```python
from build123d import *

# Parameters (mm, degrees)
SKETCH1_W                                        = 30
SKETCH1_H                                        = 30
BOSS_EXTRUDE1_DEPTH                              = 11
CUT_EXTRUDE1_DEPTH                               = 1.55
CUT_EXTRUDE2_DEPTH                               = 31.712375356
SKETCH7_W                                        = 5.55
SKETCH7_H                                        = 1.8
CUT_EXTRUDE3_DEPTH                               = 5.55
CBORE_FOR_M3_HEX_HEAD_MACHINE_SCREW1_D           = 3.5
CBORE_FOR_M3_HEX_HEAD_MACHINE_SCREW1_CBORE_D     = 6.5
CBORE_FOR_M3_HEX_HEAD_MACHINE_SCREW1_CBORE_DEPTH = 4
SKETCH10_W                                       = 1.7
SKETCH10_H                                       = 12.55
CUT_EXTRUDE4_DEPTH                               = 1.8
CUT_EXTRUDE4_DEPTH_BACK                          = 2
SKETCH14_W                                       = 13
SKETCH14_H                                       = 30


with BuildPart() as part:
    # Sketch1 → Boss-Extrude1 (new body)
    with BuildSketch(Plane(origin=(0, 0, 5), x_dir=(-1, 0, 0), z_dir=(0, 0, -1))):
        Rectangle(SKETCH1_W, SKETCH1_H)
    extrude(amount=-BOSS_EXTRUDE1_DEPTH)

    # Sketch2 → Cut-Extrude1 (cut)
    with BuildSketch(Plane(origin=(0, -4.95, 0), x_dir=(1, 0, 0), z_dir=(0, 1, 0))):
        with BuildLine():
            Line((7.432729441, -5), (-7.432729441, -5))
            ThreePointArc((-7.432729441, -5), (-7.633699531, -5.794473784), (-7.75, -6.605677687))
            Line((-7.75, -6.605677687), (-7.75, -8))
            ThreePointArc((-7.75, -8), (1.508365059, -14.936538374), (7.432729441, -5))
        make_face()
    extrude(amount=-CUT_EXTRUDE1_DEPTH, mode=Mode.SUBTRACT)

    # Sketch3 → Cut-Extrude2 (cut, through all)
    with BuildSketch(Plane(origin=(0, -6.5, 0), x_dir=(-1, 0, 0), z_dir=(0, 1, 0))):
        with BuildLine():
            Line((-5.125, 5), (5.125, 5))
            Line((5.125, 5), (5.125, 8))
            ThreePointArc((5.125, 8), (0, 13.125), (-5.125, 8))
            Line((-5.125, 8), (-5.125, 5))
        make_face()
    extrude(amount=-CUT_EXTRUDE2_DEPTH, mode=Mode.SUBTRACT)

    # Sketch7 → Cut-Extrude3 (cut)
    with BuildSketch(Plane(origin=(0, 0, 5), x_dir=(-1, 0, 0), z_dir=(0, 0, -1))):
        with Locations((0, -1.55)):
            Rectangle(SKETCH7_W, SKETCH7_H)
    extrude(amount=-CUT_EXTRUDE3_DEPTH, mode=Mode.SUBTRACT)

    # CBORE for M3 Hex Head Machine Screw1 (through all)
    with Locations(Plane(origin=(0, 0, 5), x_dir=(-1, 0, 0), z_dir=(0, 0, -1))):
        with Locations((-10, 10), (-10, -10), (10, -10), (10, 10)):
            CounterBoreHole(CBORE_FOR_M3_HEX_HEAD_MACHINE_SCREW1_D / 2, CBORE_FOR_M3_HEX_HEAD_MACHINE_SCREW1_CBORE_D / 2, CBORE_FOR_M3_HEX_HEAD_MACHINE_SCREW1_CBORE_DEPTH)

    # Sketch10 → Ø3.4 (3.4) Diameter Hole1 (revolve, cut)
    with BuildSketch(Plane(origin=(0, -2.45, 8), x_dir=(0, 0, 1), z_dir=(1, 0, 0))):
        with Locations((0.85, 6.275)):
            Rectangle(SKETCH10_W, SKETCH10_H)
    revolve(axis=Axis((0, 3.9, 8), (0, -1, 0)), mode=Mode.SUBTRACT)

    # Sketch12 → CSK for M3 Flat Head Machine Screw1 (revolve, cut)
    with BuildSketch(Plane(origin=(0, 15, 8), x_dir=(0, 0, 1), z_dir=(1, 0, 0))):
        Polygon((0, 0), (0, 30), (1.7, 30), (1.7, 4.931333959), (3.25, 4), (3.25, 0), align=None)
    revolve(axis=Axis((0, 21.35, 8), (0, -1, 0)), mode=Mode.SUBTRACT)

    # Sketch14 → Cut-Extrude4 (cut, two sides: drawn at the far end of the back side and taken through both)
    with BuildSketch(Plane(origin=(0, -6.5, 0), x_dir=(-1, 0, 0), z_dir=(0, 1, 0)).offset(-CUT_EXTRUDE4_DEPTH_BACK)):
        with Locations((-0.068435325, 5)):
            Rectangle(SKETCH14_W, SKETCH14_H)
    extrude(amount=CUT_EXTRUDE4_DEPTH + CUT_EXTRUDE4_DEPTH_BACK, mode=Mode.SUBTRACT)


solid = part.part
```
Could you check a few things on this model? Use its own coordinates, in mm. A direction names the side the tool comes from. Coordinates: 2 decimals unless noted, no trailing zeros. Write each loop counter-clockwise with the first axis right and the second up, starting at its lowest first coordinate (ties: lowest second). Pieces come first, ordered by that corner, then holes. Notation, with made-up numbers: M -19,35 L -11,35 A25 ccw -11,61 Z; hole C -12,62.25 d3. An arc over 180 degrees is marked long. Answer as CSV lines item,"result". Start each with the question number.
1) I want a section at D-D, the plane x = 0. Please give me the cut outline in (y, z) (3 decimals).
2) For faces 1 (the cylindrical face through (-7.605, -7.803, 6.972)), 2 (the flat face through (-5.125, -12, 6)), 3 (the flat face through (-7, -4.95, 8)), 4 (the flat face through (2, -8.5, 13)), which set-ups out of +Z, -Z, +X, -X, +Y, -Y let a thin tool reach every point of the face, with its end or its side?
3) We'd pull the mould along X, two halves only. Please class faces 5 (the flat face through (15, 0, 10)), 6 (the cylindrical face through (12.395, 12.197, 6.972)), 7 (the flat face through (0, 4, 5)): +X half, -X half, draft (parallel to the pull), parting line (faces both ways), or undercut.
4) Please list where these lines run through material, in increasing order: line 1 (Y direction, x = 10, z = 11.5); line 2 (Y direction, x = 10, z = 6.45); line 3 (X direction, y = 1.5, z = 8). Write a range as from..to.
5) I want a section at A-A, the plane y = -10. Please give me the cut outline in (x, z) (3 decimals).
6) I want a section at B-B, the plane x = 10. Please give me the cut outline in (y, z), and give its area (3 significant figures).
7) I want a section at C-C, the plane z = 13.5. Please give me the cut outline in (x, y).
8) For P1, Ø3, axis at x = 0.5, z = 6.5, coming from the -Y side; P2, Ø2, axis at x = -9, y = -9.5, coming from the -Z side, each with a flat end and sliding along its axis, tell me the tip position at first contact or that it passes through.
Data:
1,outline,"M -15,13.125 L -8.5,13.125 L -8.5,16 L -15,16 Z; M -4.7,5 L -2.45,5 L -2.45,6.3 L -4.7,6.3 Z; M -4.7,9.7 L -2.45,9.7 L -2.45,10.55 L -0.65,10.55 L -0.65,9.7 L 10.069,9.7 L 11,11.25 L 15,11.25 L 15,16 L -4.7,16 Z; M -0.65,5 L 10.85,5 L 10.069,6.3 L -0.65,6.3 Z"
2,face 1,"-Z"
2,face 2,"-Z, -Y"
2,face 3,"none"
2,face 4,"+Z, -Z"
3,face 5,"+X half"
3,face 6,"undercut"
3,face 7,"draft"
4,line 1,"y = -15..-11.75, -8.25..8.25, 11.75..15"
4,line 2,"y = -15..-13.25, -6.75..6.75, 13.25..15"
4,line 3,"x = -15..-1.7, 1.7..15"
5,outline,"M -15,5 L -13.25,5 L -13.25,9 L -11.75,9 L -11.75,16 L -15,16 Z; M -8.25,9 L -6.75,9 L -6.75,5 L -5.125,5 L -5.125,8 A5.125 cw 5.125,8 L 5.125,5 L 6.75,5 L 6.75,9 L 8.25,9 L 8.25,16 L -8.25,16 Z; M 11.75,9 L 13.25,9 L 13.25,5 L 15,5 L 15,16 L 11.75,16 Z"
6,outline,"M -15,5 L -13.25,5 L -13.25,9 L -11.75,9 L -11.75,16 L -15,16 Z; M -8.25,9 L -6.75,9 L -6.75,5 L 6.75,5 L 6.75,9 L 8.25,9 L 8.25,16 L -8.25,16 Z; M 11.75,9 L 13.25,9 L 13.25,5 L 15,5 L 15,16 L 11.75,16 Z"
6,area,"229 mm^2"
7,outline,"M -15,-15 L 15,-15 L 15,15 L -15,15 Z; hole C -10,-10 d3.5; hole C -10,10 d3.5; hole M -6.43,-8.5 L 6.57,-8.5 L 6.57,-4.7 L -6.43,-4.7 Z; hole C 10,-10 d3.5; hole C 10,10 d3.5"
8,P1,"stops at y = -4.7"
8,P2,"stops at z = 9"
